Check sheet for the modelled part. Datum: model origin and axes. Units: mm. Give positions to 0.01 mm unless a question says otherwise; leave off trailing zeros. Write each loop counter-clockwise with the first axis right and the second up, starting at its lowest first coordinate (ties: lowest second). Pieces come first, ordered by that corner, then holes. Notation, with made-up numbers: (86.5, 60) -> (116.5, 60) arc R20 ccw to (116.5, 72) -> close; hole circle Ø10 at (75.5, 15). An arc over 180 degrees is marked (long way). Return JSON: item names as keys, results as strings.
from build123d import *

# Parameters (mm, degrees)
F0_R     = 12.7
F1_DEPTH = 4.699
F2_DEPTH = 5.334
F3_R     = 12.7
F4_DEPTH = 1.905
F5_R     = 2.54


with BuildPart() as f1:
    # F0 (on Top) → F1 (new body)
    with BuildSketch(Plane.XY):
        Circle(F0_R)
        Polygon((-3.6661742094, 6.35), (3.6661742094, 6.35), (7.3323484187, 0), (3.6661742094, -6.35), (-3.6661742094, -6.35), (-7.3323484187, 0), align=None, mode=Mode.SUBTRACT)
        Polygon((7.3323484187, 0), (3.6661742094, 6.35), (-3.6661742094, 6.35), (-7.3323484187, 0), (-3.6661742094, -6.35), (3.6661742094, -6.35), align=None)
    extrude(amount=-F1_DEPTH)

    # F0 (on Top) → F2 (join)
    with BuildSketch(Plane.XY):
        Circle(F0_R)
        Polygon((-3.6661742094, 6.35), (3.6661742094, 6.35), (7.3323484187, 0), (3.6661742094, -6.35), (-3.6661742094, -6.35), (-7.3323484187, 0), align=None, mode=Mode.SUBTRACT)
    extrude(amount=F2_DEPTH)

    # F3 (on face) → F4 (join)
    with BuildSketch(Plane.XY.offset(5.334)):
        Circle(F3_R)
        Polygon((3.6661742094, 6.35), (5.4992612609, 3.175000092), (7.3323484187, 0), (5.4992613458, -3.174999945), (3.6661742094, -6.35), (0, -6.35), (-3.6661742094, -6.35), (-5.4992613297, -3.1749999728), (-7.3323484187, 0), (-5.4992612781, 3.1750000622), (-3.6661742094, 6.35), (0, 6.35), align=None, mode=Mode.SUBTRACT)
        with BuildLine():
            ThreePointArc((-5.4992612781, 3.1750000622), (-3.1749999689, 5.499261332), (0, 6.35))
            Line((0, 6.35), (-3.6661742094, 6.35))
            Line((-3.6661742094, 6.35), (-5.4992612781, 3.1750000622))
        make_face()
        with BuildLine():
            ThreePointArc((0, 6.35), (3.174999954, 5.4992613406), (5.4992612609, 3.175000092))
            Line((5.4992612609, 3.175000092), (3.6661742094, 6.35))
            Line((3.6661742094, 6.35), (0, 6.35))
        make_face()
        with BuildLine():
            ThreePointArc((5.4992612609, 3.175000092), (6.1336289832, 1.6435009877), (6.35, 0))
            ThreePointArc((6.35, 0), (6.1336290052, -1.6435009057), (5.4992613458, -3.174999945))
            Line((5.4992613458, -3.174999945), (7.3323484187, 0))
            Line((7.3323484187, 0), (5.4992612609, 3.175000092))
        make_face()
        with BuildLine():
            Line((3.6661742094, -6.35), (5.4992613458, -3.174999945))
            ThreePointArc((5.4992613458, -3.174999945), (3.1750000275, -5.4992612981), (0, -6.35))
            Line((0, -6.35), (3.6661742094, -6.35))
        make_face()
        with BuildLine():
            Line((-3.6661742094, -6.35), (0, -6.35))
            ThreePointArc((0, -6.35), (-3.1750000136, -5.4992613062), (-5.4992613297, -3.1749999728))
            Line((-5.4992613297, -3.1749999728), (-3.6661742094, -6.35))
        make_face()
        with BuildLine():
            ThreePointArc((-5.4992613297, -3.1749999728), (-6.35, 5.16e-08), (-5.4992612781, 3.1750000622))
            Line((-5.4992612781, 3.1750000622), (-7.3323484187, 0))
            Line((-7.3323484187, 0), (-5.4992613297, -3.1749999728))
        make_face()
    extrude(amount=F4_DEPTH)

    # F5
    f5_edges = [f1.edges().sort_by_distance(p)[0] for p in [
        (-12.7, 0, 7.239),
    ]]
    fillet(f5_edges, radius=F5_R)


solid = f1.part
(1) Thickness scan on L1, parallel to Z at x = 0.5, y = -4; L2, parallel to X at y = 5.5, z = 0.75; L3, parallel to Y at x = -6.75, z = 1.75. Record the ranges inside material, lowest first.
Reply:
{"L1": "-4.7 to 0", "L2": "-11.45 to -4.16, 4.16 to 11.45", "L3": "-10.76 to -1.01, 1.01 to 10.76"}
(2) Depth check by flat-ended pin: pin 1 Ø3 at (y, z) = (-2.5, 4) entering from +X; pin 2 Ø2.5 at (x, z) = (1.5, 3) entering from +Y; pin 3 Ø1.5 at (y, z) = (10, 3.5) entering from +X. Enter the tip coordinate at first touch or a pass-through.
Reply:
{"pin 1": "x = 12.66", "pin 2": "y = 12.7", "pin 3": "x = 8.7"}
(3) Cross-section at A-A on z = -1.5. Enter the section's corners in (x, y), then the cut area to 3 significant figures.
Reply:
{"outline": "circle Ø25.4 at (0, 0)", "area": "507 mm^2"}
(4) Release check for a two-part mould opening along Z. For faces 1 (the flat face through (4.4, -5, 7.239)), 2 (the flat face through (-3, -6, 5.334)), 3 (the flat face through (0, 0, -4.699)) record: pulls with the +Z half, pulls with the -Z half, needs draft (parallel to the pull), parting line crosses it, or undercut.
Reply:
{"face 1": "pulls with the +Z half", "face 2": "undercut", "face 3": "pulls with the -Z half"}
